```python
from build123d import *

# Parameters (mm, degrees)
SKETCH1_R             = 12.7
BOSS_EXTRUDE1_DEPTH   = 27.94
F_3_0MM_DOWEL_HOLE2_D = 3.5
SKETCH8_R             = 11.2
SKETCH8_R_2           = 2.75
CUT_EXTRUDE1_DEPTH    = 2.54


# Read off the part's stored shape, not the designer's step: CBORE for #2 Button Head Cap Screw1
with BuildPart() as part:
    # Sketch1 → Boss-Extrude1 (new body)
    with BuildSketch(Plane(origin=(0, 0, 0), x_dir=(1, 0, 0), z_dir=(0, 1, 0))):
        with Locations(Location((0, 0, 0), (0, 0, 270))):
            Circle(SKETCH1_R)
    extrude(amount=BOSS_EXTRUDE1_DEPTH)

    # Ø3.0mm Dowel Hole2 (through all)
    with Locations(Plane(origin=(0, 27.94, 0), x_dir=(1, 0, 0), z_dir=(0, 1, 0))):
        with Locations((0, 0)):
            Hole(F_3_0MM_DOWEL_HOLE2_D / 2)

    # CBORE for #2 Button Head Cap Screw1 outl → CBORE for #2 Button Head Cap Screw1 (revolve, cut)
    with BuildSketch(Plane(origin=(0, 5.08, 0), x_dir=(0, 1, 0), z_dir=(0, 0, -1))):
        Polygon((1.35255, 11.5316), (2.57937, 11.5316), (2.57937, 12.700038915), (0, 12.700038915), (0, 1.110061146), (1.35255, 1.110061146), align=None)
    revolve(axis=Axis((0, 5.08, 0), (1, 0, 0)), mode=Mode.SUBTRACT)

    # Sketch8 → Cut-Extrude1 (cut)
    with BuildSketch(Plane.XZ):
        with Locations(Location((0, 0, 0), (0, 0, 270))):
            Circle(SKETCH8_R)
        with Locations(Location((0, 0, 0), (0, 0, 270))):
            Circle(SKETCH8_R_2, mode=Mode.SUBTRACT)
    extrude(amount=-CUT_EXTRUDE1_DEPTH, mode=Mode.SUBTRACT)


solid = part.part
```
Could you check a few things on this model? Use its own coordinates, in mm. A direction names the side the tool comes from. Round coordinates to 2 decimals unless told otherwise and drop trailing zeros. Write each loop counter-clockwise with the first axis right and the second up, starting at its lowest first coordinate (ties: lowest second). Pieces come first, ordered by that corner, then holes. Notation, with made-up numbers: M 86,-18 L 105,-18 A27 ccw 105,20 Z; hole C -13.75,-1 d6. An arc over 180 degrees is marked long. Answer in a Markdown table with one row per item. Add a question column.
Q1. On a 3-axis mill with a long thin cutter (end or side, diameter ignored), from which of +Z, -Z, +X, -X, +Y, -Y can I reach the whole of each face in a straight line? I mean faces 1 (the cylindrical face through (11.99, 7.46, -0.99)), 2 (the cylindrical face through (-2.685, 1.252, 0.596)), 3 (the flat face through (-9, 0, 7)). Say none if no direction works.
Q2. Imagine slicing it at A-A (x = 0). Please give me the cut outline in (y, z).
Q3. Imagine slicing it at B-B (z = 0). Please give me the cut outline in (x, y), then the cut area to 3 significant figures.
Q4. Imagine slicing it at D-D (y = 5.75). Please give me the cut outline in (x, z), then the cut area to 3 significant figures.
Q5. Imagine slicing it at C-C (x = 8). Please give me the cut outline in (y, z).
Q6. Will these pins go through, and if not, where does the flat tip stop? pin 1 Ø4 at (x, y) = (7, 22.5) entering from +Z; pin 2 Ø1 at (x, z) = (6, 0.5) entering from -Y; pin 3 Ø5 at (y, z) = (19.5, 8.5) entering from -X.
Q7. If I drill on line 1 (Y direction, x = 12.2, z = 0); line 2 (Y direction, x = 10.5, z = 2.25); line 3 (Y direction, x = 9.75, z = -1), over which ranges is the centre line in solid material (lowest first)? Write a range as from..to.
Q8. If we mould it in two halves opening along X, with no side actions, what happens to faces 4 (the cylindrical face through (-1.669, 13.774, -0.526)), 5 (the flat face through (-2.3, 2.54, -2.3)), 6 (the flat face through (0, 0, 2)), 7 (the cylindrical face through (-12.4, 13.77, -2.75))? For each: +X half, -X half, draft (parallel to the pull), parting line (faces both ways), or undercut.
Values:
| question | item | result |
|---|---|---|
| 1 | face 1 | +X |
| 1 | face 2 | -Y |
| 1 | face 3 | +Z, -Z, +X, -X, -Y |
| 2 | outline | M 0,-12.7 L 27.94,-12.7 L 27.94,-1.75 L 0,-1.75 L 0,-2.75 L 2.54,-2.75 L 2.54,-11.2 L 0,-11.2 Z; M 0,1.75 L 27.94,1.75 L 27.94,12.7 L 0,12.7 L 0,11.2 L 2.54,11.2 L 2.54,2.75 L 0,2.75 Z |
| 3 | outline | M -12.7,0 L -11.2,0 L -11.2,2.54 L -2.75,2.54 L -2.75,0 L -1.75,0 L -1.75,27.94 L -12.7,27.94 Z; M 1.75,0 L 2.75,0 L 2.75,2.54 L 11.2,2.54 L 11.2,0 L 12.7,0 L 12.7,2.5 L 11.53,2.5 L 11.53,3.73 L 1.75,3.73 Z; M 1.75,6.43 L 11.53,6.43 L 11.53,7.66 L 12.7,7.66 L 12.7,27.94 L 1.75,27.94 Z |
| 3 | area | 536 mm^2 |
| 4 | outline | M 1.3,-1.17 A1.75 cw long 1.3,1.17 L 11.53,1.17 L 11.53,2.49 L 12.45,2.49 A12.7 ccw long 12.45,-2.49 L 11.53,-2.49 L 11.53,-1.17 Z |
| 4 | area | 468 mm^2 |
| 5 | outline | M 0,-9.86 L 27.94,-9.86 L 27.94,9.86 L 0,9.86 L 0,7.84 L 2.54,7.84 L 2.54,-7.84 L 0,-7.84 Z; hole C 5.08,0 d2.71 |
| 6 | pin 1 | z = 11.67 |
| 6 | pin 2 | y = 2.54 |
| 6 | pin 3 | x = -11.19 |
| 7 | line 1 | 0..2.5, 7.66..27.94 |
| 7 | line 2 | 2.54..27.94 |
| 7 | line 3 | 2.54..4.17, 5.99..27.94 |
| 8 | face 4 | undercut |
| 8 | face 5 | undercut |
| 8 | face 6 | draft |
| 8 | face 7 | parting line |
